Could you check a few things on this drawing? It's one solid part, dimensions in mm from its lowest x, y, z. Give positions to 0.01 mm unless a question says otherwise; leave off trailing zeros. Loops run counter-clockwise (first coordinate to the right, second up) from the corner with the lowest first, then second, coordinate; pieces in that order, holes last. Notation, with made-up numbers: M 7,0 L 25,0 A22 ccw 25,22 Z; hole C 43.5,60 d11. An arc over 180 degrees is marked long. Answer as a JSON object with one key per item and string values.
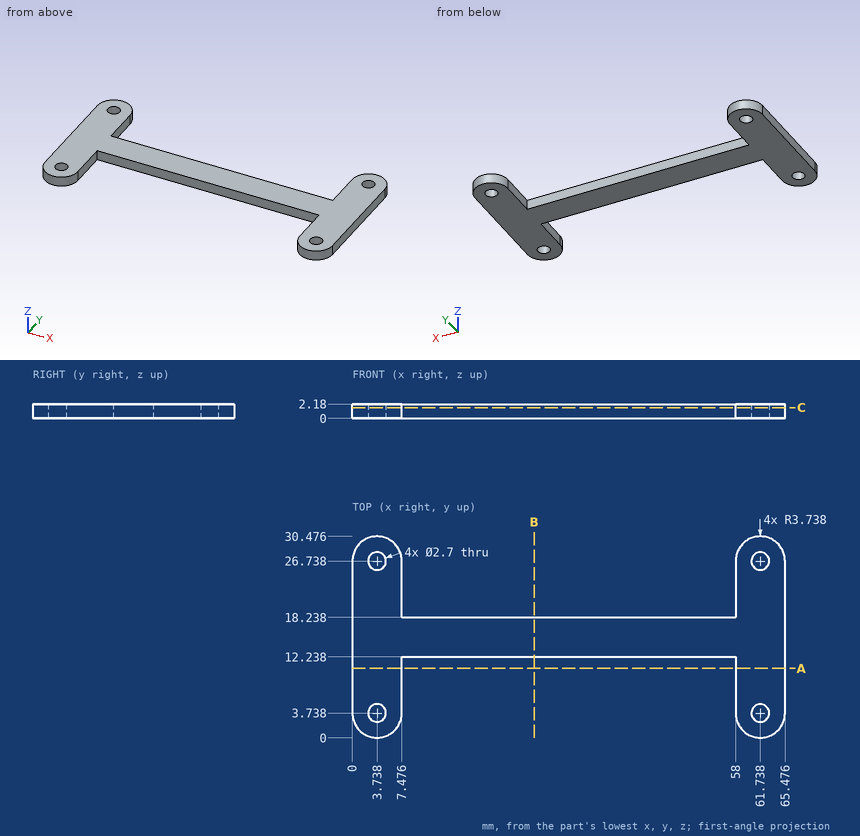
1) Please list where these lines run through material, in increasing order: line 1 along X through (y, z) = (6.5, 1.3) (1 decimal); line 2 along X through (y, z) = (4, 1.6) (1 decimal); line 3 along Y through (x, z) = (15.5, 2.05). Write a range as from..to.
Answer list:
{"line 1": "0..7.5, 58..65.5", "line 2": "0..2.4, 5.1..7.5, 58..60.4, 63.1..65.5", "line 3": "12.24..18.24"}
2) Suppose I cut it at A-A, the plane y = 10.5. Write out the boundary of the cut face in (x, z) (1 decimal), and give its area (3 significant figures).
Answer list:
{"outline": "M 0,0 L 7.5,0 L 7.5,2.2 L 0,2.2 Z; M 58,0 L 65.5,0 L 65.5,2.2 L 58,2.2 Z", "area": "32.6 mm^2"}
3) Suppose I cut it at C-C, the plane z = 1.65. Give the number of separate pieces and of enclosed holes in the cut face, and give its area (3 significant figures).
Answer list:
{"separate pieces": "1", "enclosed holes": "4", "area": "712 mm^2"}
4) Will these pins go through, and if not, where does the flat tip stop? pin 1 Ø1.1 at (x, z) = (23.5, 1.5) entering from +Y; pin 2 Ø1.6 at (x, y) = (61.74, 3.74) entering from +Z.
Answer list:
{"pin 1": "y = 18.24", "pin 2": "through"}
5) Suppose I cut it at B-B, the plane x = 27.5. Write out the boundary of the cut face in (y, z), and give its area (3 significant figures).
Answer list:
{"outline": "M 12.24,0 L 18.24,0 L 18.24,2.18 L 12.24,2.18 Z", "area": "13.1 mm^2"}
